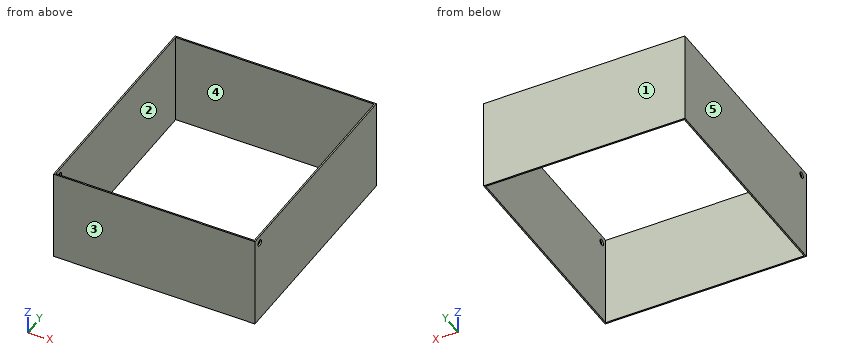
from build123d import *

# Parameters (mm, degrees)
SKETCH1_W           = 270
SKETCH1_H           = 300
BOSS_EXTRUDE1_DEPTH = 125
SKETCH5_R           = 4.2
CUT_EXTRUDE1_DEPTH  = 299


with BuildPart() as part:
    # Sketch1 → Boss-Extrude1 (new body)
    with BuildSketch(Plane.XY):
        Polygon((270, 302), (272, 302), (272, 300), (272, 0), (272, -2), (270, -2), (0, -2), (-2, -2), (-2, 0), (-2, 300), (-2, 302), (0, 302), align=None)
        with Locations((135, 150)):
            Rectangle(SKETCH1_W, SKETCH1_H, mode=Mode.SUBTRACT)
    extrude(amount=-BOSS_EXTRUDE1_DEPTH)

    # Sketch5 → Cut-Extrude1 (cut)
    with BuildSketch(Plane(origin=(272, 0, 0), x_dir=(0, 0, -1), z_dir=(1, 0, 0))):
        with Locations((10, 10)):
            Circle(SKETCH5_R)
    extrude(amount=-CUT_EXTRUDE1_DEPTH, mode=Mode.SUBTRACT)


solid = part.part
Read the model definition and answer for the solid it produces. Units are mm, in the model's axes. Face numbers are marked on the shaded views. A direction names the side the tool comes from. Give positions to 0.01 mm unless a question says otherwise; leave off trailing zeros. Write each loop counter-clockwise with the first axis right and the second up, starting at its lowest first coordinate (ties: lowest second). Pieces come first, ordered by that corner, then holes. Notation, with made-up numbers: (17, 76.25) - (31, 76.25) arc R14 cw to (31, 99.25) - close; hole circle Ø11 at (-34.75, 34). An arc over 180 degrees is marked (long way). Use CSV: the item, a comma, the result in double quotes. Start each with the question number.
Item 1: The mould has two halves that part along Y. Classify the marked faces 3, 4 and 5: pulls with the +Y half, pulls with the -Y half, needs draft (parallel to the pull), parting line crosses it, or undercut.
Item 2: The part is cut by section B-B, the plane x = 177. Give the vertices of the cut face in (y, z), and give its area (3 significant figures).
Item 3: The part is cut by section A-A, the plane y = 10. Give the vertices of the cut face in (x, z), and give its area (3 significant figures).
Item 4: For the marked faces 1 and 2, determine the directions among +Z, -Z, +X, -X, +Y, -Y from which every point of the face is accessible in a straight line to the end or side of a thin tool.
Item 5: Consider line 1 (Y direction, x = 72.5, z = -81.5); line 2 (Y direction, x = 270.95, z = -10); line 3 (X direction, y = 47, z = -7). Determine where each line is inside the solid, lowest interval first.
Item 6: The part is cut by section D-D, the plane y = 97. Give the vertices of the cut face in (x, z), and give its area (3 significant figures).
Item 7: The part is cut by section C-C, the plane z = -10. Give the vertices of the cut face in (x, y).
Taken from the geometry:
1,face 3,"pulls with the -Y half"
1,face 4,"undercut"
1,face 5,"needs draft"
2,outline,"(-2, -125) - (0, -125) - (0, 0) - (-2, 0) - close; (300, -125) - (302, -125) - (302, 0) - (300, 0) - close"
2,area,"500 mm2"
3,outline,"(-2, -125) - (0, -125) - (0, -14.2) - (-2, -14.2) - close; (-2, -5.8) - (0, -5.8) - (0, 0) - (-2, 0) - close; (270, -125) - (272, -125) - (272, -14.2) - (270, -14.2) - close; (270, -5.8) - (272, -5.8) - (272, 0) - (270, 0) - close"
3,area,"466 mm2"
4,face 1,"+Z, -Z, +X, -X, +Y"
4,face 2,"+Z, -Z"
5,line 1,"-2 to 0, 300 to 302"
5,line 2,"-2 to 5.8, 14.2 to 302"
5,line 3,"-2 to 0, 270 to 272"
6,outline,"(-2, -125) - (0, -125) - (0, 0) - (-2, 0) - close; (270, -125) - (272, -125) - (272, 0) - (270, 0) - close"
6,area,"500 mm2"
7,outline,"(-2, -2) - (272, -2) - (272, 5.8) - (270, 5.8) - (270, 0) - (0, 0) - (0, 5.8) - (-2, 5.8) - close; (-2, 14.2) - (0, 14.2) - (0, 300) - (270, 300) - (270, 14.2) - (272, 14.2) - (272, 302) - (-2, 302) - close"
